Could you check a few things on this model? Use its own coordinates, in mm. Round coordinates to 2 decimals unless told otherwise and drop trailing zeros. Write each loop counter-clockwise with the first axis right and the second up, starting at its lowest first coordinate (ties: lowest second). Pieces come first, ordered by that corner, then holes.
Autodesk Inventor part; units mm, degrees
ref_plane "YZ Plane" through (0, 0, 0) normal (1, 0, 0) x (0, 1, 0)
ref_plane "XZ Plane" through (0, 0, 0) normal (0, 1, 0) x (-1, 0, 0)
ref_plane "XY Plane" through (0, 0, 0) normal (0, 0, 1) x (1, 0, 0)
sketch "Sketch1" plane through (0, 0, 0) normal (0, 0, 1) x (1, 0, 0)
  line L0 (0, 0) -> (100, 0)
  line L1 (100, 0) -> (100, 20)
  line L2 (100, 20) -> (0, 20)
  line L3 (0, 20) -> (0, 0)
  dimension "d0" = 100
  dimension "d1" = 20
extrude "Extrusion1" add sketch "Sketch1" along normal blind 20
sketch "Sketch2" plane through (0, 20, 0) normal (0, 1, 0) x (1, 0, 0)
  circle A0 centre (10.3006, -9.5044) radius 3.7411
  circle A1 centre (23.2386, -9.5044) radius 3.8763
  circle A2 centre (92.585, -9.5044) radius 4.8406
  circle A3 centre (81.1397, -10.4639) radius 4.4927
  point P0 (0, 0)
hole "Hole1" at (10.3006, 20, 9.5044) at (23.2386, 20, 9.5044) at (81.1397, 20, 10.4639) at (92.585, 20, 9.5044) direction (0, -1, 0) diameter 5 end through all
sketch "Sketch3" plane through (0, 20, 0) normal (0, 1, 0) x (1, 0, 0)
  point P0 (0, 0)
sketch "Sketch4" plane through (0, 20, 0) normal (0, 1, 0) x (1, 0, 0)
  arc A0 (51.1615, -7.9359) -> (51.1615, -11.2858) centre (47.9614, -9.6108) ccw
  arc A1 (51.1615, -11.2858) -> (51.1615, -7.9359) centre (55.2972, -9.6108) ccw
  point P0 (0, 0)
extrude "Extrusion2" cut sketch "Sketch4" along normal mid plane 100
properties part number "measuring the torque"
Q1. If I drill on L1, parallel to Z at x = 81, y = 3.75; L2, parallel to X at y = 9, z = 10.5; L3, parallel to X at y = 6.75, z = 8.5, over which ranges is the centre line in solid material (lowest first)?
Q2. Imagine slicing it at D-D, the plane x = 55.5. Write out the boundary of the cut face in (y, z).
Q3. Imagine slicing it at B-B, the plane z = 9.25. Write out the boundary of the cut face in (x, y).
Q4. Imagine slicing it at A-A, the plane x = 80. Write out the boundary of the cut face in (y, z).
Q5. Imagine slicing it at C-C, the plane y = 6. Write out the boundary of the cut face in (x, z) (1 decimal), then the cut area to 3 significant figures.
Q6. We'd pull the mould along X, two halves only. Please class faces 1 (the flat face through (100, 10, 10)), 2 (the cylindrical face through (20.76, 9.86, 9.18)), 3 (the flat face through (49, 10, 20)), 4 (the cylindrical face through (59.756, 9.86, 9.439)): pulls with the +X half, pulls with the -X half, needs draft (parallel to the pull), parting line crosses it, or undercut.
Q7. I'm going to push flat-ended pins straight in: pin 1 Ø8 at (x, z) = (16.5, 11.5) entering from -Y; pin 2 Ø4 at (x, z) = (10.3, 9.5) entering from -Y. Where does each tip first touch, or does it pass through?
Results found:
1. L1: z = 0 to 7.97, 12.96 to 20
1. L2: x = 0 to 8.01, 12.59 to 20.95, 25.53 to 44.46, 59.67 to 78.64, 83.64 to 90.29, 94.88 to 100
1. L3: x = 0 to 8.01, 12.59 to 20.95, 25.53 to 44.52, 59.62 to 79.59, 82.69 to 90.3, 94.87 to 100
2. outline: (0, 0) - (20, 0) - (20, 5.15) - (0, 5.15) - close; (0, 14.07) - (20, 14.07) - (20, 20) - (0, 20) - close
3. outline: (0, 0) - (7.81, 0) - (7.81, 20) - (0, 20) - close; (12.79, 0) - (20.75, 0) - (20.75, 20) - (12.79, 20) - close; (25.73, 0) - (44.37, 0) - (44.37, 20) - (25.73, 20) - close; (59.74, 0) - (78.95, 0) - (78.95, 20) - (59.74, 20) - close; (83.33, 0) - (90.1, 0) - (90.1, 20) - (83.33, 20) - close; (95.07, 0) - (100, 0) - (100, 20) - (95.07, 20) - close
4. outline: (0, 0) - (20, 0) - (20, 8.24) - (0, 8.24) - close; (0, 12.69) - (20, 12.69) - (20, 20) - (0, 20) - close
5. outline: (0, 0) - (100, 0) - (100, 20) - (0, 20) - close; hole circle Ø5 at (10.3, 9.5); hole circle Ø5 at (23.2, 9.5); hole (51.2, 7.9) arc R4.5 ccw (long way) to (51.2, 11.3) arc R3.6 ccw (long way) to start; hole circle Ø5 at (81.1, 10.5); hole circle Ø5 at (92.6, 9.5)
5. area: 1,820 mm2
6. face 1: pulls with the +X half
6. face 2: undercut
6. face 3: needs draft
6. face 4: undercut
7. pin 1: stops at y = 0
7. pin 2: passes through
